Answer from the drawing. Dimensions are ordinates in mm from the lowest x, y and z of the part. Round coordinates to 2 decimals unless told otherwise and drop trailing zeros. Write each loop counter-clockwise with the first axis right and the second up, starting at its lowest first coordinate (ties: lowest second). Pieces come first, ordered by that corner, then holes. Notation, with made-up numbers: (30, -29) -> (59, -29) arc R27 cw to (59, 0) -> close; hole circle Ø11 at (2, 87.5). An arc over 180 degrees is marked (long way). Return JSON: item names as keys, results as strings. Group by question number.
(1) A cutting plane is placed at C-C on y = 16. Give the vertices of the cut face in (x, z).
(2) A cutting plane is placed at B-B on x = 12.5. Give the vertices of the cut face in (y, z), then the cut area to 3 significant figures.
(3) Straight lines are drawn through the part: line 1 (Y direction, x = 20.5, z = 17.75); line 2 (Y direction, x = 8.5, z = 15.75); line 3 (Y direction, x = 18, z = 10.25). For each, find the intervals that lie inside material, in ascending order.
(4) A cutting plane is placed at A-A on z = 12.5. Give the vertices of the cut face in (x, y), then the cut area to 3 significant figures.
(5) Given pin 1 (0.6 mm diameter, centred on y = 61, z = 10.5, fed in from -X); pin 2 (1.4 mm diameter, centred on y = 60.5, z = 11, fed in from +X); pin 3 (6 mm diameter, centred on y = 20, z = 16, fed in from +X), each flat-ended and moving along its own axis, determine where each tip first touches the part or whether it passes through.
(6) The mould has two halves that part along Y. Classify the marked faces 1, 2 and 3: released by +Y, released by -Y, zero draft, split by the parting line, or undercut.
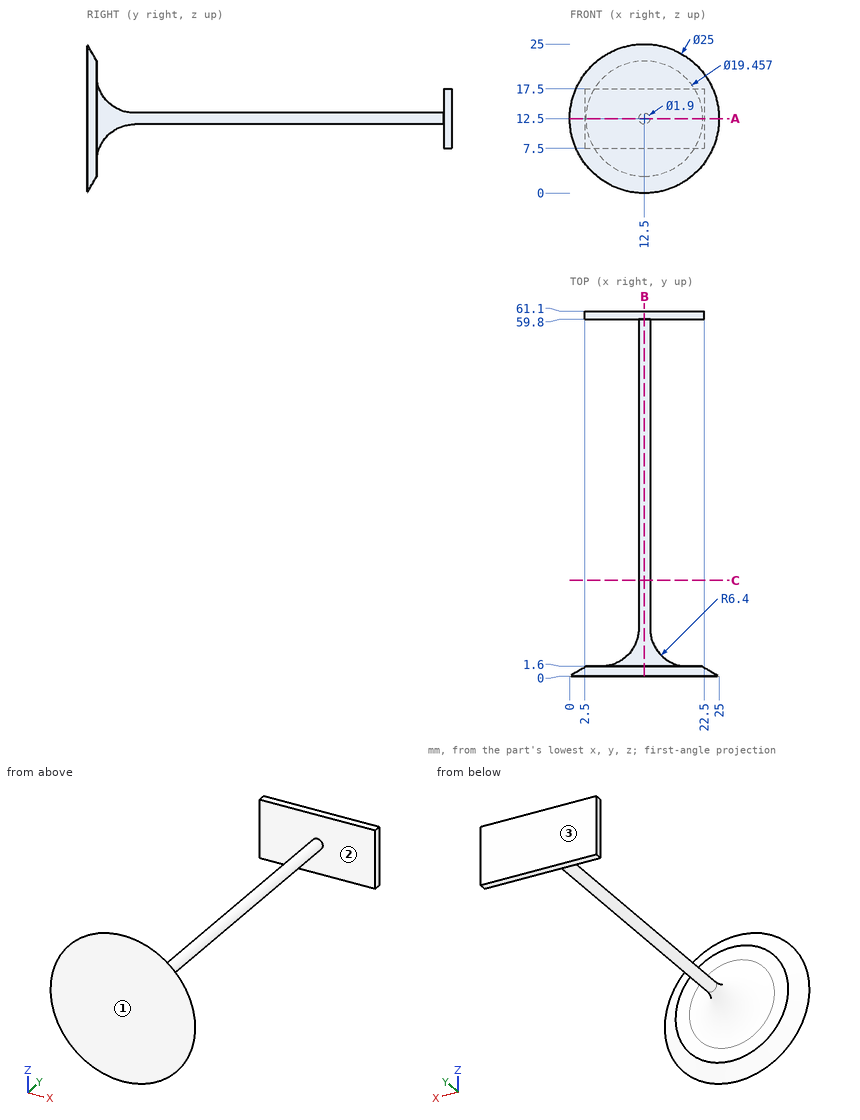
Checks:
{
 "1": {"outline": "circle Ø1.9 at (12.5, 12.5)"},
 "2": {"outline": "(0, 0) -> (1.6, 2.77) -> (1.6, 5.15) arc R6.4 cw to (8, 11.55) -> (59.8, 11.55) -> (59.8, 7.5) -> (61.1, 7.5) -> (61.1, 17.5) -> (59.8, 17.5) -> (59.8, 13.45) -> (8, 13.45) arc R6.4 cw to (1.6, 19.85) -> (1.6, 22.23) -> (0, 25) -> close", "area": "177 mm^2"},
 "3": {"line 1": "y = 0 to 1.6", "line 2": "y = 0 to 1.99, 59.8 to 61.1", "line 3": "y = 0 to 1.76, 59.8 to 61.1"},
 "4": {"outline": "(0, 0) -> (25, 0) -> (22.23, 1.6) -> (19.85, 1.6) arc R6.4 cw to (13.45, 8) -> (13.45, 59.8) -> (22.5, 59.8) -> (22.5, 61.1) -> (2.5, 61.1) -> (2.5, 59.8) -> (11.55, 59.8) -> (11.55, 8) arc R6.4 cw to (5.15, 1.6) -> (2.77, 1.6) -> close", "area": "190 mm^2"},
 "5": {"pin 1": "stops at x = 2.5", "pin 2": "stops at x = 22.5", "pin 3": "stops at x = 13.31"},
 "6": {"face 1": "released by -Y", "face 2": "undercut", "face 3": "released by +Y"}
}
